from build123d import *

# Parameters (mm, degrees)
SKETCH1_R          = 12.7
EXTRUDE1_DEPTH     = 88.9
SKETCH2_W          = 20.6375
SKETCH2_H          = 12.7
EXTRUDE2_DEPTH     = 23.8125
FILLET1_R          = 10.31875
SKETCH3_R          = 6.35
CUT_EXTRUDE1_DEPTH = 116.01434761


with BuildPart() as part:
    # Sketch1 → Extrude1 (new body)
    with BuildSketch(Plane(origin=(0, 0, 0), x_dir=(1, 0, 0), z_dir=(0, 1, 0))):
        with Locations(Location((0, 0, 0), (0, 0, 270))):
            Circle(SKETCH1_R)
    extrude(amount=EXTRUDE1_DEPTH)

    # Sketch2 → Extrude2 (add)
    with BuildSketch(Plane(origin=(0, 88.9, 0), x_dir=(-1, 0, 0), z_dir=(0, 1, 0))):
        Rectangle(SKETCH2_W, SKETCH2_H)
    extrude(amount=EXTRUDE2_DEPTH)

    # Fillet1
    fillet1_edges = [part.edges().sort_by_distance(p)[0] for p in [
        (-10.31875, 112.7125, 0),
        (10.31875, 112.7125, 0),
    ]]
    fillet(fillet1_edges, radius=FILLET1_R - 0.0001)  # a hair under: the kernel refuses the full size

    # Sketch3 → Cut-Extrude1 (cut, through all)
    with BuildSketch(Plane.XY.offset(6.35)):
        with Locations((0, 102.39375)):
            Circle(SKETCH3_R)
    extrude(amount=-CUT_EXTRUDE1_DEPTH, mode=Mode.SUBTRACT)


solid = part.part
Verification items for the finished model (mm, model axes). A direction names the side the tool comes from. Coordinates: 2 decimals unless noted, no trailing zeros. Order: outer loops, then holes, each group sorted by start corner. A loop starts at its lowest first (then second) coordinate and runs counter-clockwise, first axis right, second up. Notation, with made-up numbers: (39, 82.5) -> (49, 82.5) arc R8 ccw to (49, 90.5) -> close; hole circle Ø9 at (-17, 60). An arc over 180 degrees is marked (long way). Use CSV: the item, a comma, the result in double quotes. Start each with the question number.
Q1. Draft check along Y on faces 5 (the flat face through (0, 95, -6.35)), 6 (the cylindrical face through (-1.4, 96.2, 0.1)), 7 (the cylindrical face through (-7.376, 109.61, 0.089)). Enter one of: +Y half, -Y half, draft (parallel to the pull), parting line (faces both ways), or undercut.
Q2. Thickness scan on line 1 along Y through (x, z) = (-0.25, -3.75); line 2 along X through (y, z) = (17.5, -0.5); line 3 along Y through (x, z) = (4.75, -6). Record the ranges inside material, lowest first.
Q3. Section check B-B, the plane y = 98. Record the cut outline in (x, z).
Q4. Section check D-D, the plane y = 86.5. Record the cut outline in (x, z).
Q5. Section check A-A, the plane x = 3. Record the cut outline in (y, z).
Q6. Depth check by flat-ended pin: P1, Ø2, axis at y = 63.5, z = -9, coming from the -X side; P2, Ø10, axis at x = -8.5, z = 7, coming from the +Y side; P3, Ø2, axis at y = 96.5, z = -5, coming from the +X side. Enter the tip coordinate at first touch or a pass-through.
Q7. Tool access check on faces 1 (the flat face through (0, 95, 6.35)), 2 (the flat face through (10.319, 96, 0)), 3 (the cylindrical face through (-7.7, 43.8, -10.1)), 4 (the flat face through (-10.319, 96, 0)). Record the directions out of +Z, -Z, +X, -X, +Y, -Y that give a thin tool (end or side, any length) a straight path to the whole face; none if there is none.
Returned:
1,face 5,"draft"
1,face 6,"undercut"
1,face 7,"+Y half"
2,line 1,"y = 0 to 96.05, 108.74 to 112.71"
2,line 2,"x = -12.69 to 12.69"
2,line 3,"y = 0 to 98.18, 106.61 to 111.55"
3,outline,"(-10.32, -6.35) -> (-4.58, -6.35) -> (-4.58, 6.35) -> (-10.32, 6.35) -> close; (4.58, -6.35) -> (10.32, -6.35) -> (10.32, 6.35) -> (4.58, 6.35) -> close"
4,outline,"circle Ø25.4 at (0, 0)"
5,outline,"(0, -12.34) -> (88.9, -12.34) -> (88.9, -6.35) -> (96.8, -6.35) -> (96.8, 6.35) -> (88.9, 6.35) -> (88.9, 12.34) -> (0, 12.34) -> close; (107.99, -6.35) -> (112.27, -6.35) -> (112.27, 6.35) -> (107.99, 6.35) -> close"
6,P1,"stops at x = -9.86"
6,P2,"stops at y = 112.09"
6,P3,"stops at x = 10.32"
7,face 1,"+Z, +X, -X, +Y"
7,face 2,"+Z, -Z, +X, +Y"
7,face 3,"+Y, -Y"
7,face 4,"+Z, -Z, -X, +Y"
